Source: three-view drawing plus pictorial views. Frame: mm from the lowest corner of the part. A direction names the side the tool comes from. Give positions to 0.01 mm unless a question says otherwise; leave off trailing zeros. Order: outer loops, then holes, each group sorted by start corner. A loop starts at its lowest first (then second) coordinate and runs counter-clockwise, first axis right, second up. Notation, with made-up numbers: (31.25, -8) -> (78.25, -8) arc R13 ccw to (78.25, 11) -> close; hole circle Ø5 at (71.25, 25.25). An arc over 180 degrees is marked (long way). Answer in a Markdown table with one row per item.
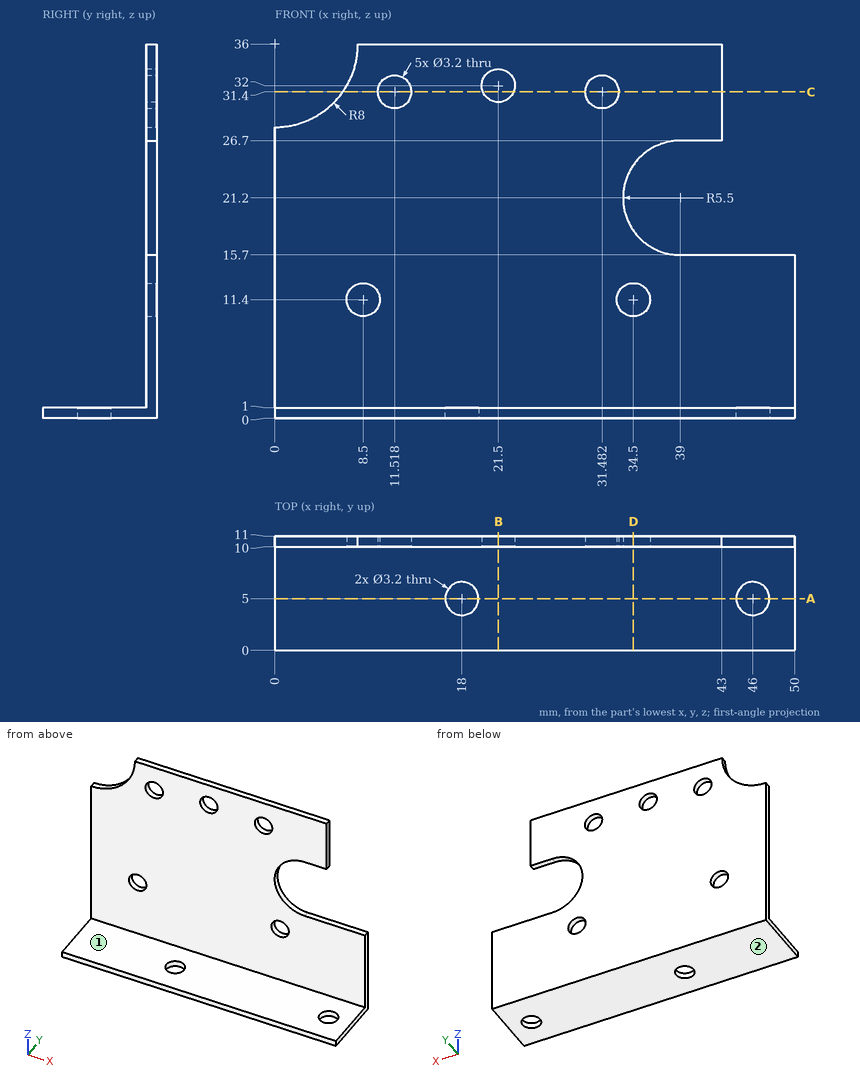
(1) Section query A-A (y = 5). Return the cut outline in (x, z), plus the area to 3 significant figures.
A:
| item | result |
|---|---|
| outline | (0, 0) -> (16.4, 0) -> (16.4, 1) -> (0, 1) -> close; (19.6, 0) -> (44.4, 0) -> (44.4, 1) -> (19.6, 1) -> close; (47.6, 0) -> (50, 0) -> (50, 1) -> (47.6, 1) -> close |
| area | 43.6 mm^2 |
(2) Section query C-C (z = 31.4). Return the cut outline in (x, y), plus the area to 3 significant figures.
A:
| item | result |
|---|---|
| outline | (6.55, 10) -> (9.92, 10) -> (9.92, 11) -> (6.55, 11) -> close; (13.12, 10) -> (20.02, 10) -> (20.02, 11) -> (13.12, 11) -> close; (22.98, 10) -> (29.88, 10) -> (29.88, 11) -> (22.98, 11) -> close; (33.08, 10) -> (43, 10) -> (43, 11) -> (33.08, 11) -> close |
| area | 27.1 mm^2 |
(3) First-contact query: pin 1 Ø5 at (x, y) = (19.5, 3.5) entering from +Z; pin 2 Ø5 at (x, z) = (7, 32.5) entering from -Y; pin 3 Ø0.8 at (y, z) = (10.5, 30) entering from +X. Flat tips, straight axial feed; report the tip coordinate or a pass-through.
A:
| item | result |
|---|---|
| pin 1 | stops at z = 1 |
| pin 2 | stops at y = 10 |
| pin 3 | stops at x = 43 |
(4) Access query for the marked faces 1 and 2. Directions: +Z, -Z, +X, -X, +Y, -Y. A direction counts if a zero-diameter tool reaches every point of the face in a straight line with its end or side. Return the directions, or none.
A:
| item | result |
|---|---|
| face 1 | +Z, +X, -X, -Y |
| face 2 | -Z, +X, -X, +Y, -Y |
(5) Section query B-B (x = 21.5). Return the cut outline in (y, z).
A:
| item | result |
|---|---|
| outline | (0, 0) -> (11, 0) -> (11, 30.4) -> (10, 30.4) -> (10, 1) -> (0, 1) -> close; (10, 33.6) -> (11, 33.6) -> (11, 36) -> (10, 36) -> close |
(6) Section query D-D (x = 34.5). Return the cut outline in (y, z), plus the area to 3 significant figures.
A:
| item | result |
|---|---|
| outline | (0, 0) -> (11, 0) -> (11, 9.8) -> (10, 9.8) -> (10, 1) -> (0, 1) -> close; (10, 13) -> (11, 13) -> (11, 18.04) -> (10, 18.04) -> close; (10, 24.36) -> (11, 24.36) -> (11, 36) -> (10, 36) -> close |
| area | 36.5 mm^2 |
(7) Ray query, probe 1 along Y at (x, z) = (46, 0.35); probe 2 along Z at (x, y) = (34.5, 10.6); probe 3 along Z at (x, y) = (19, 6.75). Return the intervals inside material, ascending.
A:
| item | result |
|---|---|
| probe 1 | y = 0 to 3.4, 6.6 to 11 |
| probe 2 | z = 0 to 9.8, 13 to 18.04, 24.36 to 36 |
| probe 3 | z = 0 to 1 |
